For this review, take the finished solid that the model builds, in its own axes (mm). Coordinates: 2 decimals unless noted, no trailing zeros. Loops run counter-clockwise (first coordinate to the right, second up) from the corner with the lowest first, then second, coordinate; pieces in that order, holes last. Notation, with made-up numbers: (57.25, 86.5) -> (68.25, 86.5) arc R28 ccw to (68.25, 125.5) -> close; hole circle Ø3 at (-39, -34.75). An arc over 180 degrees is marked (long way). Answer in a Markdown table with one row per item.
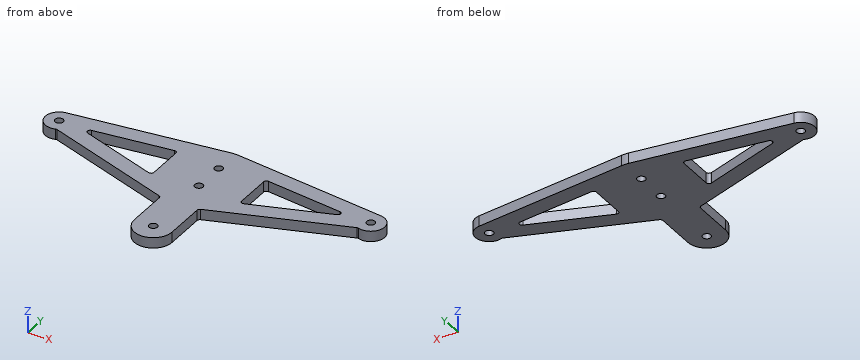
from build123d import *

# Parameters (mm, degrees)
ESBO_O2_R                = 1.5
RESSALTO_EXTRUS_O1_DEPTH = 3.8
FILETE1_R                = 10


with BuildPart() as part:
    # Esboço2 → Ressalto-extrusão1 (new body)
    with BuildSketch(Plane.XY):
        with BuildLine():
            Line((-0.609346717, 4.962730758), (56.5, 11.974876818))
            Line((56.5, 11.974876818), (113.609346717, 4.962730758))
            ThreePointArc((113.609346717, 4.962730758), (117.879129474, -1.092746803), (111.434372539, -4.748558798))
            ThreePointArc((111.434372539, -4.748558798), (111.114278546, -4.698294837), (110.794916153, -4.753014958))
            Line((110.794916153, -4.753014958), (64.023669106, -20.899867583))
            ThreePointArc((64.023669106, -20.899867583), (63.535650292, -21.264748688), (63.35, -21.845123182))
            Line((63.35, -21.845123182), (63.35, -36.675123182))
            ThreePointArc((63.35, -36.675123182), (56.5, -43.525123182), (49.65, -36.675123182))
            Line((49.65, -36.675123182), (49.65, -21.845123182))
            ThreePointArc((49.65, -21.845123182), (49.464349708, -21.264748688), (48.976330894, -20.899867583))
            Line((48.976330894, -20.899867583), (2.205083847, -4.753014958))
            ThreePointArc((2.205083847, -4.753014958), (1.885721454, -4.698294837), (1.565627461, -4.748558798))
            ThreePointArc((1.565627461, -4.748558798), (-4.879129474, -1.092746803), (-0.609346717, 4.962730758))
        make_face()
        with Locations(Location((0, 0, 0), (0, 0, 180))):
            Circle(ESBO_O2_R, mode=Mode.SUBTRACT)
        with Locations(Location((113, 0, 0), (0, 0, 180))):
            Circle(ESBO_O2_R, mode=Mode.SUBTRACT)
        with Locations(Location((56.5, 2.174876818, 0), (0, 0, 180))):
            Circle(ESBO_O2_R, mode=Mode.SUBTRACT)
        with Locations(Location((56.5, -9.525123182, 0), (0, 0, 180))):
            Circle(ESBO_O2_R, mode=Mode.SUBTRACT)
        with Locations(Location((56.5, -36.675123182, 0), (0, 0, 180))):
            Circle(ESBO_O2_R, mode=Mode.SUBTRACT)
        with BuildLine():
            Line((72.4, 2.847248961), (72.4, -10.257469431))
            ThreePointArc((72.4, -10.257469431), (72.819625506, -11.071819139), (73.726330894, -11.20272503))
            Line((73.726330894, -11.20272503), (101.726975538, -1.536053496))
            ThreePointArc((101.726975538, -1.536053496), (102.395124292, -0.485868251), (101.522513987, 0.401748255))
            Line((101.522513987, 0.401748255), (73.521869343, 3.839795112))
            ThreePointArc((73.521869343, 3.839795112), (72.737379952, 3.596204682), (72.4, 2.847248961))
        make_face(mode=Mode.SUBTRACT)
        with BuildLine():
            Line((11.477486013, 0.401748255), (39.478130657, 3.839795112))
            ThreePointArc((39.478130657, 3.839795112), (40.262620048, 3.596204682), (40.6, 2.847248961))
            Line((40.6, 2.847248961), (40.6, -10.257469431))
            ThreePointArc((40.6, -10.257469431), (40.180374494, -11.071819139), (39.273669106, -11.20272503))
            Line((39.273669106, -11.20272503), (11.273024462, -1.536053496))
            ThreePointArc((11.273024462, -1.536053496), (10.604875708, -0.485868251), (11.477486013, 0.401748255))
        make_face(mode=Mode.SUBTRACT)
    extrude(amount=RESSALTO_EXTRUS_O1_DEPTH)

    # Filete1
    filete1_edges = [part.edges().sort_by_distance(p)[0] for p in [
        (56.5, 11.974876818, 1.9),
    ]]
    fillet(filete1_edges, radius=FILETE1_R)


solid = part.part
Item 1: For L1, parallel to Y at x = 56.5, z = 2.2; L2, parallel to Y at x = 101.5, z = 0.75; L3, parallel to Y at x = 0, z = 1.1, list the stretches that pass through material, from the lowest coordinate up.
Worked answers:
| item | result |
|---|---|
| L1 | -43.53 to -38.18, -35.18 to -11.03, -8.03 to 0.67, 3.67 to 11.9 |
| L2 | -7.96 to -1.61, 0.4 to 6.45 |
| L3 | -5 to -1.5, 1.5 to 5.04 |
Item 2: Take a section at B-B, the plane y = -6.5. State the section outline as (x, z) points, and give its area (3 significant figures).
Worked answers:
| item | result |
|---|---|
| outline | (7.27, 0) -> (25.65, 0) -> (25.65, 3.8) -> (7.27, 3.8) -> close; (40.6, 0) -> (72.4, 0) -> (72.4, 3.8) -> (40.6, 3.8) -> close; (87.35, 0) -> (105.73, 0) -> (105.73, 3.8) -> (87.35, 3.8) -> close |
| area | 261 mm² |
Item 3: Take a section at D-D, the plane z = 1.95. Count the separate pieces of the cut face and the enclosed holes in it, and give its area (3 significant figures).
Worked answers:
| item | result |
|---|---|
| separate pieces | 1 |
| enclosed holes | 7 |
| area | 2,320 mm² |
Item 4: Insertion check: pin 1 (1.9 mm diameter, centred on y = -29.5, z = 2, fed in from -X); pin 2 (4 mm diameter, centred on x = 113, y = 0, fed in from -Z); pin 3 (1.5 mm diameter, centred on y = 5, z = 1.5, fed in from -X). Each pin has a flat end and moves straight along its axis. Give the tip position at first contact, or say it passes through.
Worked answers:
| item | result |
|---|---|
| pin 1 | x = 49.65 |
| pin 2 | z = 0 |
| pin 3 | x = -2.63 |
Item 5: Take a section at A-A, the plane x = 90.5. State the section outline as (y, z) points, and give its area (3 significant figures).
Worked answers:
| item | result |
|---|---|
| outline | (-11.76, 0) -> (-5.41, 0) -> (-5.41, 3.8) -> (-11.76, 3.8) -> close; (1.76, 0) -> (7.8, 0) -> (7.8, 3.8) -> (1.76, 3.8) -> close |
| area | 47.1 mm² |
Item 6: Take a section at C-C, the plane x = 56.5. State the section outline as (y, z) points, and give its area (3 significant figures).
Worked answers:
| item | result |
|---|---|
| outline | (-43.53, 0) -> (-38.18, 0) -> (-38.18, 3.8) -> (-43.53, 3.8) -> close; (-35.18, 0) -> (-11.03, 0) -> (-11.03, 3.8) -> (-35.18, 3.8) -> close; (-8.03, 0) -> (0.67, 0) -> (0.67, 3.8) -> (-8.03, 3.8) -> close; (3.67, 0) -> (11.9, 0) -> (11.9, 3.8) -> (3.67, 3.8) -> close |
| area | 176 mm² |
